from build123d import *

# Parameters (mm, degrees)
SKETCH1_R                = 59
EXTRUDE1_DEPTH           = 3
EXTRUDE2_DEPTH           = 3
CIRPATTERN1_COUNT        = 6
F_2_0_2_DIAMETER_HOLE1_D = 2
F_2_0_2_DIAMETER_HOLE3_D = 2
CIRPATTERN2_COUNT        = 3
CIRPATTERN2_ANGLE        = 120


with BuildPart() as part:
    # Sketch1 → Extrude1 (new, symmetric)
    with BuildSketch(Plane(origin=(0, 0, 0), x_dir=(0, 0, -1), z_dir=(1, 0, 0))):
        Circle(SKETCH1_R)
        Polygon((18.592791334, 22.158025869), (-9.893017633, 27.180842557), (-28.485808967, 5.022816688), (-18.592791334, -22.158025869), (9.893017633, -27.180842557), (28.485808967, -5.022816688), align=None, mode=Mode.SUBTRACT)
    extrude(amount=EXTRUDE1_DEPTH, both=True)

    # Sketch2 → Extrude2 (add, symmetric)
    with BuildSketch(Plane(origin=(0, 0, 0), x_dir=(0, 0, -1), z_dir=(1, 0, 0))):
        with BuildLine():
            Line((-2, 67.961805723), (-0.262709442, 61.478149092))
            ThreePointArc((-0.262709442, 61.478149092), (-0.58620663, 59.77173183), (-2.122608272, 58.961805723))
            ThreePointArc((-2.122608272, 58.961805723), (28.679663449, 51.560419941), (51.21368579, 29.294340542))
            ThreePointArc((51.21368579, 29.294340542), (36.791707484, 48.186627241), (17.927108603, 62.644803614))
            ThreePointArc((17.927108603, 62.644803614), (8.312130826, 66.609702921), (-2, 67.961805723))
        make_face()
    extrude2 = extrude(amount=EXTRUDE2_DEPTH, both=True)

    # CirPattern1: Extrude2 ×6 about axis
    cirpattern1_axis = Axis((0, 0, 0), (1, 0, 0))
    for i in range(1, CIRPATTERN1_COUNT):
        add(extrude2.rotate(cirpattern1_axis, i * 360 / CIRPATTERN1_COUNT))

    # Ø2.0 (2) Diameter Hole1 (through all)
    with Locations(Plane(origin=(3, 0, 0), x_dir=(0, 0, -1), z_dir=(1, 0, 0))):
        with Locations((-9.893017633, 27.180842557), (18.592791334, 22.158025869), (28.485808967, -5.022816688), (9.893017633, -27.180842557), (-18.592791334, -22.158025869), (-28.485808967, 5.022816688)):
            Hole(F_2_0_2_DIAMETER_HOLE1_D / 2)

    # Ø2.0 (2) Diameter Hole3 (through all)
    with Locations(Plane(origin=(3, 0, 0), x_dir=(0, 0, -1), z_dir=(1, 0, 0))):
        with Locations((-0.069478726, 25.448687602)):
            f_2_0_2_diameter_hole3 = Hole(F_2_0_2_DIAMETER_HOLE3_D / 2)

    # CirPattern2: Ø2.0 (2) Diameter Hole3 ×3 about axis
    cirpattern2_axis = Axis((0, 0, 0), (-1, 0, 0))
    for i in range(1, CIRPATTERN2_COUNT):
        add(f_2_0_2_diameter_hole3.rotate(cirpattern2_axis, i * CIRPATTERN2_ANGLE / (CIRPATTERN2_COUNT - 1)), mode=Mode.SUBTRACT)


solid = part.part
CAD build for the part. Positions are in the model's coordinates, mm. A direction names the side the tool comes from. Coordinates: 2 decimals unless noted, no trailing zeros. Write each loop counter-clockwise with the first axis right and the second up, starting at its lowest first coordinate (ties: lowest second). Pieces come first, ordered by that corner, then holes. Notation, with made-up numbers: M -1,69 L 28,69 A20 cw 28,74 Z; hole C 12.25,12.25 d2. An arc over 180 degrees is marked long. Return JSON: item names as keys, results as strings.
Item 1: Probe line 1 (Y direction, x = -2.3, z = 0); line 2 (Y direction, x = 0.2, z = -54.5); line 3 (Z direction, x = -0.3, y = 20). List the from-to ranges inside material, lowest first. Write a range as from..to.
Findings below:
{"line 1": "y = -67.91..-25.44, 26.45..67.91", "line 2": "y = -39.5..-30.81, -23.03..32.36", "line 3": "z = -62.99..-19.38, 15.92..55.87"}
Item 2: Which spindle directions (+Z, -Z, +X, -X, +Y, -Y) get a long thin tool onto all of the face, cutting with end or side? Do faces 1 (the cylindrical face through (0.042, -7.046, -60.318)), 2 (the flat face through (0.042, 33.373, -55.517)), 3 (the flat face through (0.04, -8.89, -25.24)), 4 (the flat face through (0.042, -33.373, 55.517)). Say none if no direction does.
Findings below:
{"face 1": "-Z, +X, -X", "face 2": "+X, -X, +Y", "face 3": "+X, -X", "face 4": "+X, -X, -Y"}
Item 3: Drop flat-ended pins along their axis: pin 1 Ø3 at (x, z) = (-1.5, 48.5) entering from +Y; pin 2 Ø2 at (x, y) = (-1, 11) entering from +Z; pin 3 Ø1.5 at (x, z) = (0.5, -12.5) entering from -Y. Give the stop position or say it passes through.
Findings below:
{"pin 1": "stops at y = 45.8", "pin 2": "stops at z = 59.5", "pin 3": "stops at y = -58.25"}
Item 4: Slice it at D-D, the plane y = -44.5. Write the cut outline in (x, z).
Findings below:
{"outline": "M -3,-48.88 L 3,-48.88 L 3,40.27 L -3,40.27 Z"}
Item 5: Two-plate mould, pull along Z, no slides. Class faces 5 (the flat face through (0.042, 16.246, 19.068)), 6 (the cylindrical face through (0.042, -40.607, -53.426)), 7 (the flat face through (0.042, 31.392, 56.66)): +Z half, -Z half, draft (parallel to the pull), parting line (faces both ways), or undercut.
Findings below:
{"face 5": "undercut", "face 6": "-Z half", "face 7": "+Z half"}
Item 6: Slice it at B-B, the plane z = 3.5. Write the cut outline in (x, y), and give its area (3 significant figures).
Findings below:
{"outline": "M -3,-67.58 L 3,-67.58 L 3,-24.82 L -3,-24.82 Z; M -3,26.05 L 3,26.05 L 3,58.94 L -3,58.94 Z", "area": "454 mm2"}
Item 7: Slice it at A-A, the plane y = -19. Write the cut outline in (x, z).
Findings below:
{"outline": "M -3,-56.3 L 3,-56.3 L 3,-16.76 L -3,-16.76 Z; M -3,19.74 L 3,19.74 L 3,63.08 L -3,63.08 Z"}
Item 8: Slice it at C-C, the plane z = -47.5. Write the cut outline in (x, y).
Findings below:
{"outline": "M -3,-45.47 L 3,-45.47 L 3,35.24 L -3,35.24 Z"}
